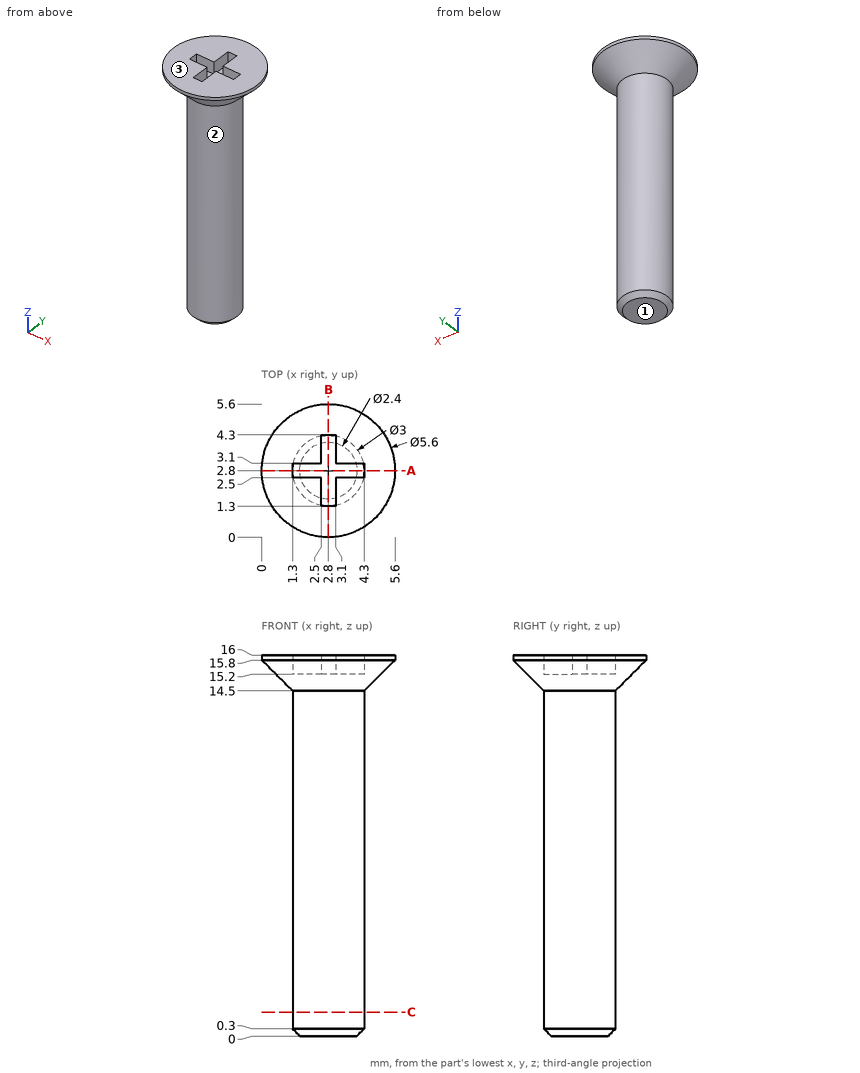
Verification items for this drawing (mm, ordinates from the low corner). Coordinates: 2 decimals unless noted, no trailing zeros. Loops run counter-clockwise (first coordinate to the right, second up) from the corner with the lowest first, then second, coordinate; pieces in that order, holes last. Notation, with made-up numbers: (-11, 73.25) -> (31, 73.25) arc R23 cw to (31, 83.25) -> close; hole circle Ø11 at (15.5, -10.5). An arc over 180 degrees is marked (long way). Put each result on its own line as item: value.
1. Thickness scan on line 1 (Y direction, x = 2.7, z = 7.75); line 2 (Z direction, x = 0.9, y = 1.75); line 3 (Z direction, x = 2.6, y = 0.7). Record the ranges inside material, lowest first.
Result set:
line 1: y = 1.3 to 4.3
line 2: z = 15.17 to 16
line 3: z = 15.11 to 16
2. Gauge pin test, flat ends, axial feed: P1, Ø1.5, axis at x = 4.5, z = 12.5, coming from the +Y side; P2, Ø0.9, axis at x = 2, z = 16, coming from the +Y side; P3, Ø2, axis at x = 4, z = 14, coming from the -Y side. Record the tip position at first contact, or that the pin passes through.
Result set:
P1: stops at y = 3.96
P2: stops at y = 5.58
P3: stops at y = 1.06
3. Section check A-A, the plane y = 2.8. Record the boundary of the cut face in (x, z), then the cut area to 3 significant figures.
Result set:
outline: (0, 15.8) -> (1.3, 14.5) -> (1.3, 0.3) -> (1.6, 0) -> (4, 0) -> (4.3, 0.3) -> (4.3, 14.5) -> (5.6, 15.8) -> (5.6, 16) -> (4.3, 16) -> (4.3, 15.2) -> (1.3, 15.2) -> (1.3, 16) -> (0, 16) -> close
area: 47.7 mm^2
4. Mould release check, pull along Z, two halves, no side actions. Record for the marked faces 1, 2 and 3: pulls with the +Z half, pulls with the -Z half, needs draft (parallel to the pull), parting line crosses it, or undercut.
Result set:
face 1: pulls with the -Z half
face 2: needs draft
face 3: pulls with the +Z half
5. Section check C-C, the plane z = 1. Record the boundary of the cut face in (x, y).
Result set:
outline: circle Ø3 at (2.8, 2.8)
